Read the model definition and answer for the solid it produces. Units are mm, in the model's axes. A direction names the side the tool comes from. Give positions to 0.01 mm unless a question says otherwise; leave off trailing zeros. Write each loop counter-clockwise with the first axis right and the second up, starting at its lowest first coordinate (ties: lowest second). Pieces come first, ordered by that corner, then holes. Notation, with made-up numbers: M 73,22.5 L 77,22.5 A18 ccw 77,41.5 Z; hole C -34,85.25 d10. An arc over 180 degrees is marked long. Use a Markdown table: item, result. Add a question column.
Item 1: A cutting plane is placed at D-D on z = -28. Determine the outline of the cut face in (x, y).
Item 2: A cutting plane is placed at A-A on y = 0.45. Determine the outline of the cut face in (x, z).
Item 3: A cutting plane is placed at B-B on z = -5.75. Determine the outline of the cut face in (x, y).
Item 4: For faces 1 (the flat face through (6.8, 2, -37)), 2 (the flat face through (3.2, 2, -38)), 3 (the flat face through (5, 1, -75.4)), determine the directions among +Z, -Z, +X, -X, +Y, -Y from which every point of the face is accessible in a straight line to the end or side of a thin tool.
Item 5: Given P1, Ø1.5, axis at y = 2, z = -50.5, coming from the +X side; P2, Ø0.9, axis at y = 1, z = -45, coming from the -X side, each flat-ended and moving along its own axis, determine where each tip first touches the part or whether it passes through.
Item 6: The mould has two halves that part along Z. Classify faces 4 (the flat face through (1, 1, -11.5)), 5 (the flat face through (-0.4, 2, -6)), 6 (the flat face through (5, 1, 0.4)): pulls with the +Z half, pulls with the -Z half, needs draft (parallel to the pull), parting line crosses it, or undercut.
Item 7: A cutting plane is placed at C-C on x = 5. Determine the outline of the cut face in (y, z).
Item 8: Consider probe 1 along X at (y, z) = (1.2, -69.25); probe 2 along Z at (x, y) = (3, 0.65); probe 3 along Z at (x, y) = (10, 0.8). Determine where each line is inside the solid, lowest interval first. Write a range as [from, to].
from build123d import *

# Parameters (mm, degrees)
BOSS_EXTRUDE1_DEPTH = 3
SKETCH2_R           = 4.25
CUT_EXTRUDE1_DEPTH  = 3
SKETCH3_W           = 10
SKETCH3_H           = 3
BOSS_EXTRUDE2_DEPTH = 0.4
SKETCH4_W           = 10
SKETCH4_H           = 3
BOSS_EXTRUDE3_DEPTH = 0.4
SKETCH5_W           = 11.9
SKETCH5_H           = 3
BOSS_EXTRUDE4_DEPTH = 0.4
SKETCH6_W           = 52
SKETCH6_H           = 3
BOSS_EXTRUDE5_DEPTH = 0.4
SKETCH7_W           = 11.9
SKETCH7_H           = 3
BOSS_EXTRUDE6_DEPTH = 0.4
SKETCH8_W           = 52
SKETCH8_H           = 3
BOSS_EXTRUDE7_DEPTH = 0.4
SKETCH9_W           = 52
SKETCH9_H           = 3
CUT_EXTRUDE2_DEPTH  = 0.1
SKETCH10_W          = 52
SKETCH10_H          = 3
CUT_EXTRUDE3_DEPTH  = 0.1


with BuildPart() as part:
    # Sketch1 → Boss-Extrude1 (new body)
    with BuildSketch(Plane(origin=(0, 0, 0), x_dir=(1, 0, 0), z_dir=(0, 1, 0))):
        Polygon((0, 11.5), (3.5, 11.5), (3.5, 63.5), (0, 63.5), (0, 75), (10, 75), (10, 63.5), (6.5, 63.5), (6.5, 11.5), (10, 11.5), (10, 0), (0, 0), align=None)
    extrude(amount=BOSS_EXTRUDE1_DEPTH)

    # Sketch2 → Cut-Extrude1 (cut)
    with BuildSketch(Plane(origin=(0, 3, 0), x_dir=(1, 0, 0), z_dir=(0, 1, 0))):
        with Locations(Location((5, 69.25, 0), (0, 0, 270))):
            Circle(SKETCH2_R)
        with Locations(Location((5, 5.75, 0), (0, 0, 90))):
            Circle(SKETCH2_R)
    extrude(amount=-CUT_EXTRUDE1_DEPTH, mode=Mode.SUBTRACT)

    # Sketch3 → Boss-Extrude2 (add)
    with BuildSketch(Plane.XY):
        with Locations((5, 1.5)):
            Rectangle(SKETCH3_W, SKETCH3_H)
    extrude(amount=BOSS_EXTRUDE2_DEPTH)

    # Sketch4 → Boss-Extrude3 (add)
    with BuildSketch(Plane(origin=(0, 0, -75), x_dir=(-1, 0, 0), z_dir=(0, 0, -1))):
        with Locations((-5, 1.5)):
            Rectangle(SKETCH4_W, SKETCH4_H)
    extrude(amount=BOSS_EXTRUDE3_DEPTH)

    # Sketch5 → Boss-Extrude4 (add)
    with BuildSketch(Plane(origin=(10, 0, 0), x_dir=(0, 0, -1), z_dir=(1, 0, 0))):
        with Locations((69.45, 1.5)):
            Rectangle(SKETCH5_W, SKETCH5_H)
        with Locations((5.55, 1.5)):
            Rectangle(SKETCH5_W, SKETCH5_H)
    extrude(amount=BOSS_EXTRUDE4_DEPTH)

    # Sketch6 → Boss-Extrude5 (add)
    with BuildSketch(Plane(origin=(6.5, 0, 0), x_dir=(0, 0, -1), z_dir=(1, 0, 0))):
        with Locations((37.5, 1.5)):
            Rectangle(SKETCH6_W, SKETCH6_H)
    extrude(amount=BOSS_EXTRUDE5_DEPTH)

    # Sketch7 → Boss-Extrude6 (add)
    with BuildSketch(Plane.ZY):
        with Locations((-5.55, 1.5)):
            Rectangle(SKETCH7_W, SKETCH7_H)
        with Locations((-69.45, 1.5)):
            Rectangle(SKETCH7_W, SKETCH7_H)
    extrude(amount=BOSS_EXTRUDE6_DEPTH)

    # Sketch8 → Boss-Extrude7 (add)
    with BuildSketch(Plane.ZY.offset(-3.5)):
        with Locations((-37.5, 1.5)):
            Rectangle(SKETCH8_W, SKETCH8_H)
    extrude(amount=BOSS_EXTRUDE7_DEPTH)

    # Sketch9 → Cut-Extrude2 (cut)
    with BuildSketch(Plane.ZY.offset(-3.1)):
        with Locations((-37.5, 1.5)):
            Rectangle(SKETCH9_W, SKETCH9_H)
    extrude(amount=-CUT_EXTRUDE2_DEPTH, mode=Mode.SUBTRACT)

    # Sketch10 → Cut-Extrude3 (cut)
    with BuildSketch(Plane(origin=(6.9, 0, 0), x_dir=(0, 0, -1), z_dir=(1, 0, 0))):
        with Locations((37.5, 1.5)):
            Rectangle(SKETCH10_W, SKETCH10_H)
    extrude(amount=-CUT_EXTRUDE3_DEPTH, mode=Mode.SUBTRACT)


solid = part.part
Filled in:
| question | item | result |
|---|---|---|
| 1 | outline | M 3.2,0 L 6.8,0 L 6.8,3 L 3.2,3 Z |
| 2 | outline | M -0.4,-75.4 L 10.4,-75.4 L 10.4,-63.5 L 6.8,-63.5 L 6.8,-11.5 L 10.4,-11.5 L 10.4,0.4 L -0.4,0.4 L -0.4,-11.5 L 3.2,-11.5 L 3.2,-63.5 L -0.4,-63.5 Z; hole C 5,-69.25 d8.5; hole C 5,-5.75 d8.5 |
| 3 | outline | M -0.4,0 L 0.75,0 L 0.75,3 L -0.4,3 Z; M 9.25,0 L 10.4,0 L 10.4,3 L 9.25,3 Z |
| 4 | face 1 | +X, +Y, -Y |
| 4 | face 2 | -X, +Y, -Y |
| 4 | face 3 | -Z, +X, -X, +Y, -Y |
| 5 | P1 | x = 6.8 |
| 5 | P2 | x = 3.2 |
| 6 | face 4 | undercut |
| 6 | face 5 | needs draft |
| 6 | face 6 | pulls with the +Z half |
| 7 | outline | M 0,-75.4 L 3,-75.4 L 3,-73.5 L 0,-73.5 Z; M 0,-65 L 3,-65 L 3,-10 L 0,-10 Z; M 0,-1.5 L 3,-1.5 L 3,0.4 L 0,0.4 Z |
| 8 | probe 1 | [-0.4, 0.75], [9.25, 10.4] |
| 8 | probe 2 | [-75.4, -73], [-65.5, -63.5], [-11.5, -9.5], [-2, 0.4] |
| 8 | probe 3 | [-75.4, -63.5], [-11.5, 0.4] |
